```python
from build123d import *

# Parameters (mm, degrees)
ESQUISSE1_W             = 64.5
ESQUISSE1_H             = 62.4
BOSS_EXTRU_1_DEPTH      = 9.5
ENL_V_MAT_EXTRU_1_DEPTH = 46.866681807
CONG_1_R                = 5


with BuildPart() as part:
    # Esquisse1 → Boss.-Extru.1 (new body)
    with BuildSketch(Plane(origin=(0, 0, 0), x_dir=(1, 0, 0), z_dir=(0, 1, 0))):
        Rectangle(ESQUISSE1_W, ESQUISSE1_H)
    extrude(amount=BOSS_EXTRU_1_DEPTH)

    # Esquisse2 → Enlèv. mat.-Extru.1 (cut, through all)
    with BuildSketch(Plane(origin=(0, 9.5, 0), x_dir=(1, 0, 0), z_dir=(0, 1, 0))):
        Polygon((-26.95, 25.9), (-11.35, 25.9), (-11.35, 22.45), (-12.25, 21.55), (-12.25, 16.55), (-11.35, 15.65), (-11.35, 12.2), (-26.95, 12.2), (-26.95, 15.65), (-26.05, 16.55), (-26.05, 21.55), (-26.95, 22.45), align=None)
        Polygon((-7.55, 25.9), (8.05, 25.9), (8.05, 22.45), (7.15, 21.55), (7.15, 16.55), (8.05, 15.65), (8.05, 12.2), (-7.55, 12.2), (-7.55, 15.65), (-6.65, 16.55), (-6.65, 21.55), (-7.55, 22.45), align=None)
        Polygon((11.85, 25.9), (27.45, 25.9), (27.45, 22.45), (26.55, 21.55), (26.55, 16.55), (27.45, 15.65), (27.45, 12.2), (11.85, 12.2), (11.85, 15.65), (12.75, 16.55), (12.75, 21.55), (11.85, 22.45), align=None)
        Polygon((-7.55, 6.8), (8.05, 6.8), (8.05, 3.35), (7.15, 2.45), (7.15, -2.55), (8.05, -3.45), (8.05, -6.9), (-7.55, -6.9), (-7.55, -3.45), (-6.65, -2.55), (-6.65, 2.45), (-7.55, 3.35), align=None)
        Polygon((11.85, 6.8), (27.45, 6.8), (27.45, 3.35), (26.55, 2.45), (26.55, -2.55), (27.45, -3.45), (27.45, -6.9), (11.85, -6.9), (11.85, -3.45), (12.75, -2.55), (12.75, 2.45), (11.85, 3.35), align=None)
        Polygon((-7.55, -12.3), (8.05, -12.3), (8.05, -15.75), (7.15, -16.65), (7.15, -21.65), (8.05, -22.55), (8.05, -26), (-7.55, -26), (-7.55, -22.55), (-6.65, -21.65), (-6.65, -16.65), (-7.55, -15.75), align=None)
        Polygon((11.85, -12.3), (27.45, -12.3), (27.45, -15.75), (26.55, -16.65), (26.55, -21.65), (27.45, -22.55), (27.45, -26), (11.85, -26), (11.85, -22.55), (12.75, -21.65), (12.75, -16.65), (11.85, -15.75), align=None)
        Polygon((-26.95, 6.8), (-11.35, 6.8), (-11.35, 3.35), (-12.25, 2.45), (-12.25, -2.55), (-11.35, -3.45), (-11.35, -6.9), (-26.95, -6.9), (-26.95, -3.45), (-26.05, -2.55), (-26.05, 2.45), (-26.95, 3.35), align=None)
        Polygon((-26.95, -12.3), (-11.35, -12.3), (-11.35, -15.75), (-12.25, -16.65), (-12.25, -21.65), (-11.35, -22.55), (-11.35, -26), (-26.95, -26), (-26.95, -22.55), (-26.05, -21.65), (-26.05, -16.65), (-26.95, -15.75), align=None)
    extrude(amount=-ENL_V_MAT_EXTRU_1_DEPTH, mode=Mode.SUBTRACT)

    # Congé1
    cong_1_edges = [part.edges().sort_by_distance(p)[0] for p in [
        (32.25, 4.75, 31.2),
        (-32.25, 4.75, 31.2),
        (-32.25, 4.75, -31.2),
        (32.25, 4.75, -31.2),
    ]]
    fillet(cong_1_edges, radius=CONG_1_R)


solid = part.part
```
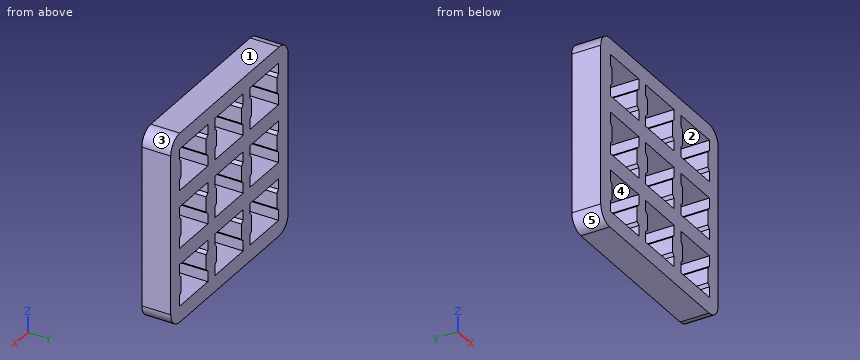
Verification items for the finished model (mm, model axes). Face numbers are marked on the shaded views. A direction names the side the tool comes from. Give positions to 0.01 mm unless a question says otherwise; leave off trailing zeros. Order: outer loops, then holes, each group sorted by start corner. A loop starts at its lowest first (then second) coordinate and runs counter-clockwise, first axis right, second up. Notation, with made-up numbers: (-8.75, -3) - (25.25, -3) arc R21 ccw to (25.25, 18) - close; hole circle Ø4 at (61, 20.5). An arc over 180 degrees is marked (long way). Answer as CSV lines item,"result". Start each with the question number.
Item 1: Access from +Z, -Z, +X, -X, +Y, -Y to the whole of each face (thin tool, end or side, straight path). Record for the marked faces 1 and 2.
Item 2: Section check C-C, the plane y = 7. State how many separate pieces and enclosed holes the cut face has, plus the area to 3 significant figures.
Item 3: Section check A-A, the plane x = -18.5. Record the boundary of the cut face in (y, z), plus the area to 3 significant figures.
Item 4: Material ranges on L1, parallel to X at y = 6.75, z = 6.5; L2, parallel to Z at x = -6.5, y = 4; L3, parallel to X at y = 1.25, z = -18, recorded low to high.
Item 5: Gauge pin test, flat end, axial feed: pin 1 (2 mm diameter, centred on x = 24, z = -14, fed in from -Y). Record the tip position at first contact, or that the pin passes through.
Item 6: Section check B-B, the plane z = -20. Record the boundary of the cut face in (x, y), plus the area to 3 significant figures.
Item 7: Mould release check, pull along X, two halves, no side actions. Record for the marked faces 3, 4 and 5: released by +X, released by -X, zero draft, split by the parting line, or undercut.
Filled in:
1,face 1,"+Z, +X, -X, +Y, -Y"
1,face 2,"+Y, -Y"
2,separate pieces,"1"
2,enclosed holes,"9"
2,area,"2,180 mm^2"
3,outline,"(0, -31.2) - (9.5, -31.2) - (9.5, -25.9) - (0, -25.9) - close; (0, -12.2) - (9.5, -12.2) - (9.5, -6.8) - (0, -6.8) - close; (0, 6.9) - (9.5, 6.9) - (9.5, 12.3) - (0, 12.3) - close; (0, 26) - (9.5, 26) - (9.5, 31.2) - (0, 31.2) - close"
3,area,"202 mm^2"
4,L1,"-32.25 to -26.95, -11.35 to -7.55, 8.05 to 11.85, 27.45 to 32.25"
4,L2,"-31.2 to -25.9, -12.2 to -6.8, 6.9 to 12.3, 26 to 31.2"
4,L3,"-32.25 to -26.05, -12.25 to -6.65, 7.15 to 12.75, 26.55 to 32.25"
5,pin 1,"through"
6,outline,"(-32.25, 0) - (-26.05, 0) - (-26.05, 9.5) - (-32.25, 9.5) - close; (-12.25, 0) - (-6.65, 0) - (-6.65, 9.5) - (-12.25, 9.5) - close; (7.15, 0) - (12.75, 0) - (12.75, 9.5) - (7.15, 9.5) - close; (26.55, 0) - (32.25, 0) - (32.25, 9.5) - (26.55, 9.5) - close"
6,area,"219 mm^2"
7,face 3,"released by +X"
7,face 4,"undercut"
7,face 5,"released by -X"
